Here's how the part is built. I have some questions about the finished solid (model axes, mm). Round coordinates to 2 decimals unless told otherwise and drop trailing zeros. Loops run counter-clockwise (first coordinate to the right, second up) from the corner with the lowest first, then second, coordinate; pieces in that order, holes last. Notation, with made-up numbers: M 86.25,23.5 L 141.25,23.5 A21 cw 141.25,35.5 Z; hole C 29.5,68 d9. An arc over 180 degrees is marked long. Use a Markdown table: item, result.
```python
from build123d import *

# Parameters (mm, degrees)
SKETCH_R  = 4
PAD_DEPTH = 6


with BuildPart() as part:
    # Sketch → Pad (new body)
    with BuildSketch(Plane.XZ):
        with BuildLine():
            Line((46.160259, -16.650643), (8.660317, 48.301296))
            ThreePointArc((8.660317, 48.301296), (0, 53.301337), (-8.660316, 48.301296))
            Line((-8.660316, 48.301296), (-46.160259, -16.650643))
            ThreePointArc((-46.160259, -16.650643), (-46.160252, -26.650639), (-37.5, -31.650635))
            Line((-37.5, -31.650635), (37.5, -31.650635))
            ThreePointArc((37.5, -31.650635), (46.160252, -26.650639), (46.160259, -16.650643))
        make_face()
        with Locations((0, 43.30127)):
            Circle(SKETCH_R, mode=Mode.SUBTRACT)
        with Locations((37.5, -21.650635)):
            Circle(SKETCH_R, mode=Mode.SUBTRACT)
        with Locations((-37.5, -21.650635)):
            Circle(SKETCH_R, mode=Mode.SUBTRACT)
        Circle(SKETCH_R, mode=Mode.SUBTRACT)
    extrude(amount=PAD_DEPTH)


solid = part.part
```
Q1. Imagine slicing it at D-D, the plane z = -13. Please give me the cut outline in (x, y).
Return value:
| item | result |
|---|---|
| outline | M -44.05,-6 L 44.05,-6 L 44.05,0 L -44.05,0 Z |
Q2. Imagine slicing it at C-C, the plane y = -1.9. Please give me the cut outline in (x, z).
Return value:
| item | result |
|---|---|
| outline | M -46.16,-16.65 A10 ccw -37.5,-31.65 L 37.5,-31.65 A10 ccw 46.16,-16.65 L 8.66,48.3 A10 ccw -8.66,48.3 Z; hole C -37.5,-21.65 d8; hole C 0,0 d8; hole C 0,43.3 d8; hole C 37.5,-21.65 d8 |
Q3. Imagine slicing it at B-B, the plane z = 2.5. Please give me the cut outline in (x, y), then the cut area to 3 significant figures.
Return value:
| item | result |
|---|---|
| outline | M -35.1,-6 L -3.12,-6 L -3.12,0 L -35.1,0 Z; M 3.12,-6 L 35.1,-6 L 35.1,0 L 3.12,0 Z |
| area | 384 mm^2 |
Q4. I need wall thicknesses on line 1 (X direction, y = -5.3, z = -20); line 2 (Z direction, x = 34.5, y = -5.65); line 3 (X direction, y = -4.65, z = -25). Which ranges of each line are inside material? Lowest first, please. Write a range as from..to.
Return value:
| item | result |
|---|---|
| line 1 | x = -47.36..-41.14, -33.86..33.86, 41.14..47.36 |
| line 2 | z = -31.65..-24.3, -19..3.55 |
| line 3 | x = -46.92..-39.69, -35.31..35.31, 39.69..46.92 |
Q5. We'd pull the mould along X, two halves only. Please class faces 1 (the flat face through (27.673, -2.958, 15.371)), 2 (the flat face through (-27.15, -2.96, 16.28)), 3 (the cylindrical face through (-0.867, -2.958, -3.905)): pulls with the +X half, pulls with the -X half, needs draft (parallel to the pull), parting line crosses it, or undercut.
Return value:
| item | result |
|---|---|
| face 1 | pulls with the +X half |
| face 2 | pulls with the -X half |
| face 3 | undercut |
Q6. Will these pins go through, and if not, where does the flat tip stop? P1, Ø1.5, axis at y = -1.5, z = 16.5, coming from the +X side; P2, Ø6.5, axis at x = 0, z = 0, coming from the -Y side; P3, Ø3, axis at x = -25, y = -5, coming from the +Z side; P4, Ø1, axis at x = 33.5, y = -3.5, coming from the +Z side.
Return value:
| item | result |
|---|---|
| P1 | stops at x = 27.45 |
| P2 | passes through |
| P3 | stops at z = 22.6 |
| P4 | stops at z = 6.14 |
Q7. Imagine slicing it at A-A, the plane x = 0. Please give me the cut outline in (y, z), then the cut area to 3 significant figures.
Return value:
| item | result |
|---|---|
| outline | M -6,-31.65 L 0,-31.65 L 0,-4 L -6,-4 Z; M -6,4 L 0,4 L 0,39.3 L -6,39.3 Z; M -6,47.3 L 0,47.3 L 0,53.3 L -6,53.3 Z |
| area | 414 mm^2 |
